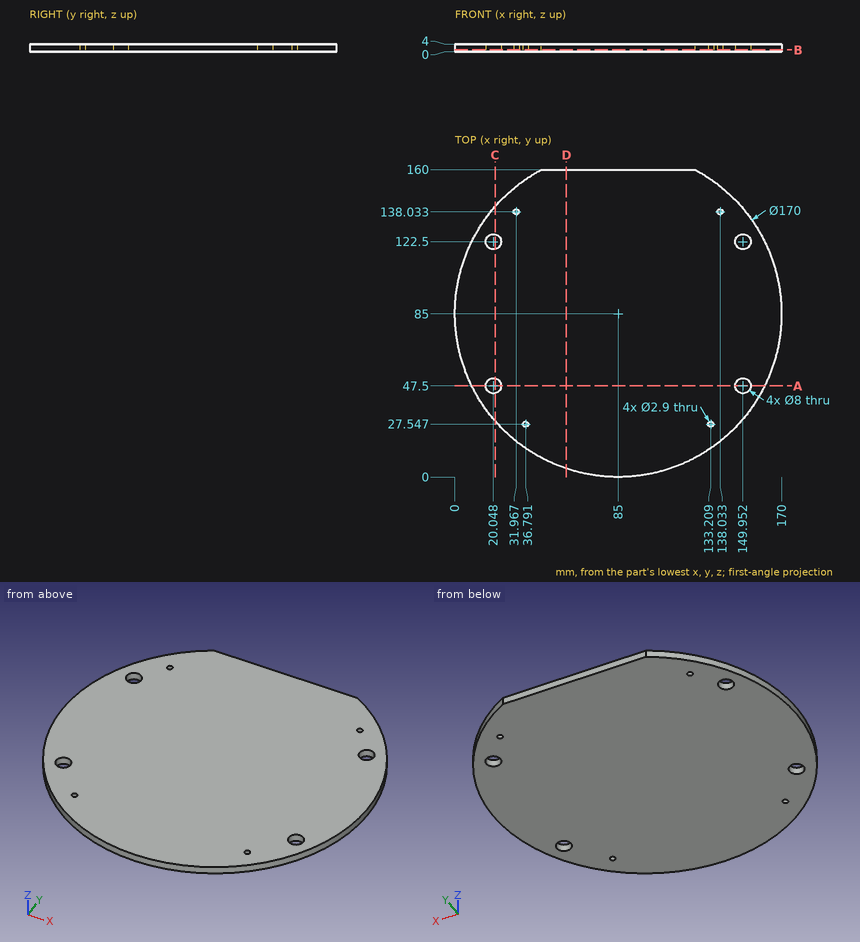
Part print with two shaded views. Sizes in mm from the minimum x, y, z corner. Round coordinates to 2 decimals unless told otherwise and drop trailing zeros. Order: outer loops, then holes, each group sorted by start corner. A loop starts at its lowest first (then second) coordinate and runs counter-clockwise, first axis right, second up. Notation, with made-up numbers: (17, 65) - (73, 65) arc R7 ccw to (73, 75) - close; hole circle Ø3 at (51, 31). An arc over 180 degrees is marked (long way). Answer as CSV lines item,"result". Start each with the question number.
1. Pin check, flat tips, straight feed: pin 1 (1.5 mm diameter, centred on y = 40, z = 2, fed in from +X); pin 2 (1 mm diameter, centred on y = 115, z = 0.5, fed in from -X). Stop position of each tip, or through.
2. Drill centre lines: L1, parallel to X at y = 125.5, z = 3.35 (1 decimal); L2, parallel to Y at x = 21.5, z = 3.5 (1 decimal); L3, parallel to X at y = 46.5, z = 2.75 (1 decimal). Where is each one in solid material? Low to high. Write a range as [from, to].
3. Saw through at C-C, the plane x = 21. Write the cut outline in (y, z) (1 decimal), and give its area (3 significant figures).
4. Saw through at A-A, the plane y = 47.5. Write the cut outline in (x, z), and give its area (3 significant figures).
5. Saw through at D-D, the plane x = 58. Write the cut outline in (y, z).
6. Saw through at B-B, the plane z = 0.95. Count the separate pieces of the cut face and the enclosed holes in it, and give its area (3 significant figures).
Model answer:
1,pin 1,"stops at x = 157.57"
1,pin 2,"stops at x = 5.28"
2,L1,"x = [10.3, 17.4], [22.7, 147.3], [152.6, 159.7]"
2,L2,"y = [28.5, 43.8], [51.2, 118.8], [126.2, 141.5]"
2,L3,"x = [9.2, 16.2], [23.9, 146.1], [153.8, 160.8]"
3,outline,"(29.1, 0) - (43.6, 0) - (43.6, 4) - (29.1, 4) - close; (51.4, 0) - (118.6, 0) - (118.6, 4) - (51.4, 4) - close; (126.4, 0) - (140.9, 0) - (140.9, 4) - (126.4, 4) - close"
3,area,"385 mm²"
4,outline,"(8.72, 0) - (16.05, 0) - (16.05, 4) - (8.72, 4) - close; (24.05, 0) - (145.95, 0) - (145.95, 4) - (24.05, 4) - close; (153.95, 0) - (161.28, 0) - (161.28, 4) - (153.95, 4) - close"
4,area,"546 mm²"
5,outline,"(4.4, 0) - (160, 0) - (160, 4) - (4.4, 4) - close"
6,separate pieces,"1"
6,enclosed holes,"8"
6,area,"21,900 mm²"
